```python
from build123d import *

# Parameters (mm, degrees)
SKETCH2_R           = 1.6
BOSS_EXTRUDE1_DEPTH = 5


with BuildPart() as part:
    # Sketch2 → Boss-Extrude1 (new body)
    with BuildSketch(Plane(origin=(0, 0, 0), x_dir=(0, 1, 0), z_dir=(0, 0, 1))):
        with BuildLine():
            Line((-10, 0), (-10, 30))
            Line((-10, 30), (-5.341066605, 38.069509349))
            Line((-5.341066605, 38.069509349), (-9.671193624, 40.569509349))
            Line((-9.671193624, 40.569509349), (10.328806376, 75.210525501))
            Line((10.328806376, 75.210525501), (14.658933395, 72.710525501))
            Line((14.658933395, 72.710525501), (21, 49.045342756))
            Line((21, 49.045342756), (10, 29.992783873))
            Line((10, 29.992783873), (10, 0))
            ThreePointArc((10, 0), (0, -10), (-10, 0))
        make_face()
        with Locations(Location((0, 0, 0), (0, 0, 270))):
            Circle(SKETCH2_R, mode=Mode.SUBTRACT)
        with Locations(Location((0, 26, 0), (0, 0, 270))):
            Circle(SKETCH2_R, mode=Mode.SUBTRACT)
    extrude(amount=BOSS_EXTRUDE1_DEPTH)


solid = part.part
```
Check sheet for the modelled part. Datum: model origin and axes. Units: mm. A direction names the side the tool comes from. Coordinates: 2 decimals unless noted, no trailing zeros. Write each loop counter-clockwise with the first axis right and the second up, starting at its lowest first coordinate (ties: lowest second). Pieces come first, ordered by that corner, then holes. Notation, with made-up numbers: (80.5, -17.5) -> (106.5, -17.5) arc R29 cw to (106.5, 20.5) -> close; hole circle Ø6 at (-17.5, 45.5). An arc over 180 degrees is marked (long way). Use a Markdown table: item, result.
1. Sectioned sample at A-A (x = -26). Enter the section's corners in (y, z), plus the area to 3 significant figures.
Reported:
| item | result |
|---|---|
| outline | (-10, 0) -> (-1.6, 0) -> (-1.6, 5) -> (-10, 5) -> close; (1.6, 0) -> (10, 0) -> (10, 5) -> (1.6, 5) -> close |
| area | 84.0 mm2 |
2. Go/stop test with flat-tipped pins: pin 1 Ø1.5 at (x, z) = (-21, 1.5) entering from +Y; pin 2 Ø3 at (y, z) = (-2, 3) entering from +X; pin 3 Ø1 at (y, z) = (9, 0.5) entering from +X. Record where each tip stops, or that it passes through.
Reported:
| item | result |
|---|---|
| pin 1 | stops at y = 10 |
| pin 2 | stops at x = 9.99 |
| pin 3 | stops at x = 5.27 |
3. Sectioned sample at D-D (y = 3.5). Enter the section's corners in (x, z).
Reported:
| item | result |
|---|---|
| outline | (-63.38, 0) -> (9.37, 0) -> (9.37, 5) -> (-63.38, 5) -> close |
4. Tool access check on faces 5 (the flat face through (-15, 10, 2)), 6 (the flat face through (-15, -10, 2)), 7 (the flat face through (-33.98, -7.7, 2.46)). Record the directions out of +Z, -Z, +X, -X, +Y, -Y that give a thin tool (end or side, any length) a straight path to the whole face; none if there is none.
Reported:
| item | result |
|---|---|
| face 5 | +Z, -Z, +X, +Y |
| face 6 | +Z, -Z, +X, -X, -Y |
| face 7 | +Z, -Z, -Y |
5. Sectioned sample at B-B (z = 1.75). Enter the section's corners in (x, y).
Reported:
| item | result |
|---|---|
| outline | (-75.21, 10.33) -> (-40.57, -9.67) -> (-38.07, -5.34) -> (-30, -10) -> (0, -10) arc R10 ccw to (0, 10) -> (-29.99, 10) -> (-49.05, 21) -> (-72.71, 14.66) -> close; hole circle Ø3.2 at (-26, 0); hole circle Ø3.2 at (0, 0) |
6. Sectioned sample at C-C (x = -4.5). Enter the section's corners in (y, z), plus the area to 3 significant figures.
Reported:
| item | result |
|---|---|
| outline | (-10, 0) -> (10, 0) -> (10, 5) -> (-10, 5) -> close |
| area | 100 mm2 |
7. Scan lines: line 1 along Y through (x, z) = (-26, 1.7); line 2 along Y through (x, z) = (-1, 0.4); line 3 along X through (y, z) = (7, 2.15). Record each from-to range of solid material in increasing order.
Reported:
| item | result |
|---|---|
| line 1 | y = -10 to -1.6, 1.6 to 10 |
| line 2 | y = -10 to -1.25, 1.25 to 10 |
| line 3 | x = -69.44 to 7.14 |
8. Release check for a two-part mould opening along X. For faces 1 (the flat face through (-39.302, -7.476, 2.465)), 2 (the cylindrical face through (10, 0, 2)), 3 (the flat face through (-33, 2, 5)), 4 (the flat face through (-73.98, 12.46, 2.46)) record: pulls with the +X half, pulls with the -X half, needs draft (parallel to the pull), parting line crosses it, or undercut.
Reported:
| item | result |
|---|---|
| face 1 | undercut |
| face 2 | pulls with the +X half |
| face 3 | needs draft |
| face 4 | pulls with the -X half |
